```python
from build123d import *

# Parameters (mm, degrees)
SKETCH1_R           = 3.937
SKETCH1_R_2         = 2.413
BOSS_EXTRUDE1_DEPTH = 29.21


with BuildPart() as part:
    # Sketch1 → Boss-Extrude1 (new body)
    with BuildSketch(Plane(origin=(0, 0, 0), x_dir=(1, 0, 0), z_dir=(0, 1, 0))):
        Circle(SKETCH1_R)
        Circle(SKETCH1_R_2, mode=Mode.SUBTRACT)
    extrude(amount=BOSS_EXTRUDE1_DEPTH)

    # Sketch2 one side → Revolve1 (revolve)
    with BuildSketch(Plane.XY):
        with BuildLine():
            ThreePointArc((0, -2.54), (4.166998508, -1.889526586), (7.9375, 0))
            Line((7.9375, 0), (0, 0))
            Line((0, 0), (0, -2.54))
        make_face()
    revolve(axis=Axis((0, 0, 0), (0, -1, 0)))

    # Sketch3 → Revolve2 (revolve)
    with BuildSketch(Plane.XY):
        Polygon((2.413, 16.51), (2.413, 29.21), (2.032, 16.51), align=None)
        Polygon((2.413, 0), (2.413, 16.51), (2.032, 16.51), (1.5367, 0), align=None)
    revolve(axis=Axis((0, 0, 0), (0, 1, 0)))


solid = part.part
```
CAD build for the part. Positions are in the model's coordinates, mm. Coordinates: 2 decimals unless noted, no trailing zeros. Loops run counter-clockwise (first coordinate to the right, second up) from the corner with the lowest first, then second, coordinate; pieces in that order, holes last. Notation, with made-up numbers: (9, 47) - (23, 47) arc R27 cw to (23, 78) - close; hole circle Ø8 at (-9.5, 15). An arc over 180 degrees is marked (long way). Return JSON: item names as keys, results as strings.
1. Drop flat-ended pins along their axis: pin 1 (5 mm diameter, centred on x = -4, y = 7, fed in from -Z); pin 2 (2 mm diameter, centred on x = -4, z = 4, fed in from -Y); pin 3 (4 mm diameter, centred on x = -3.5, z = 5, fed in from +Y); pin 4 (1.5 mm diameter, centred on x = -5.5, y = 19, fed in from -Z). Give the stop position or say it passes through.
Result:
{"pin 1": "stops at z = -3.64", "pin 2": "stops at y = -1.72", "pin 3": "stops at y = 0", "pin 4": "passes through"}
2. Band-saw the part on B-B (x = 0). Give the cut face in (y, z).
Result:
{"outline": "(0, -7.94) - (0, -3.94) - (29.21, -3.94) - (29.21, -2.41) - (0, -1.54) - (0, 1.54) - (29.21, 2.41) - (29.21, 3.94) - (0, 3.94) - (0, 7.94) arc R13.67 ccw to start"}
3. Band-saw the part on D-D (x = 3.5). Give the cut face in (y, z).
Result:
{"outline": "(0, -7.12) - (0, -1.8) - (29.21, -1.8) - (29.21, 1.8) - (0, 1.8) - (0, 7.12) arc R13.22 ccw to start"}
4. Band-saw the part on C-C (y = 17). Give the cut face in (x, z).
Result:
{"outline": "circle Ø7.87 at (0, 0); hole circle Ø4.09 at (0, 0)"}
5. Band-saw the part on A-A (z = 0). Give the cut face in (x, y), and give its area (3 significant figures).
Result:
{"outline": "(-7.94, 0) arc R13.67 ccw to (7.94, 0) - (3.94, 0) - (3.94, 29.21) - (2.41, 29.21) - (1.54, 0) - (-1.54, 0) - (-2.41, 29.21) - (-3.94, 29.21) - (-3.94, 0) - close", "area": "142 mm2"}
6. Probe L1, parallel to Z at x = 1, y = 25.5; L2, parallel to X at y = 7, z = -1; L3, parallel to Z at x = -1.75, y = 27.5. List the from-to ranges inside material, lowest first. Write a range as from..to.
Result:
{"L1": "z = -3.81..-2.07, 2.07..3.81", "L2": "x = -3.81..-1.43, 1.43..3.81", "L3": "z = -3.53..-1.59, 1.59..3.53"}
7. Mould opens along X. For faces 1 (the cylindrical face through (-0.853, 14.401, 3.843)), 2 (the conical face through (-0.43, 14.4, 1.92)), 3 (the flat face through (-2, 29.21, 2)) say: released by +X, released by -X, zero draft, split by the parting line, or undercut.
Result:
{"face 1": "split by the parting line", "face 2": "undercut", "face 3": "zero draft"}
